Autodesk Inventor part; units mm, degrees
ref_plane "YZ Plane" through (0, 0, 0) normal (1, 0, 0) x (0, 1, 0)
ref_plane "XZ Plane" through (0, 0, 0) normal (0, 1, 0) x (-1, 0, 0)
ref_plane "XY Plane" through (0, 0, 0) normal (0, 0, 1) x (1, 0, 0)
sketch "Sketch1" plane through (0, 0, 0) normal (0, 1, 0) x (-1, 0, 0)
  line L0 (0, 0) -> (254, 0)
  line L1 (254, 0) -> (254, -119.38)
  line L2 (254, -119.38) -> (0, -119.38)
  line L3 (0, -119.38) -> (0, 0)
  line L4 (186.69, 67.31) -> (67.31, 67.31)
  line L5 (67.31, 67.31) -> (67.31, -186.69)
  line L6 (67.31, -186.69) -> (186.69, -186.69)
  line L7 (186.69, -186.69) -> (186.69, 67.31)
  line L8 (186.69, 67.31) -> (254, 0)
  line L9 (67.31, 67.31) -> (0, 0)
  line L10 (186.69, -186.69) -> (254, -119.38)
  line L11 (0, -119.38) -> (67.31, -186.69)
  line L12 (62.2907, -7.1202) -> (161.0967, -7.1202)
  line L13 (164.2717, -10.2952) -> (164.2717, -109.1012)
  line L14 (161.0967, -112.2762) -> (62.2907, -112.2762)
  line L15 (59.1157, -109.1012) -> (59.1157, -10.2952)
  arc A0 (62.2907, -7.1202) -> (59.1157, -10.2952) centre (62.2907, -10.2952) ccw
  arc A1 (164.2717, -10.2952) -> (161.0967, -7.1202) centre (161.0967, -10.2952) ccw
  arc A2 (161.0967, -112.2762) -> (164.2717, -109.1012) centre (161.0967, -109.1012) ccw
  arc A3 (59.1157, -109.1012) -> (62.2907, -112.2762) centre (62.2907, -109.1012) ccw
  line L16 (254, -119.38) -> (127, -119.38)
  line L17 (126.9917, -59.69) -> (127, -119.38)
  point P0 (164.2717, -112.2762)
  point P1 (164.2717, -7.1202)
  point P2 (59.1157, -112.2762)
  point P3 (127, -59.69)
  point P4 (127, -59.69)
  dimension "d0" = 254
  dimension "d1" = 119.38
  dimension "d2" = 119.38
  dimension "d3" = 254
  dimension "d8" = 95.1907
  dimension "d14" = 105.156
  dimension "d15" = 105.156
  dimension "d22" = 3.175
  dimension "d50" = 127
  dimension "d51" = 59.69
extrude "Extrusion1" add sketch "Sketch1" along normal blind 25.4
sketch "Sketch3" plane through (0, 0, 0) normal (0, -1, 0) x (1, 0, 0)
  line L0 (-80.7772, -112.268) -> (-173.2332, -112.268)
  line L1 (-179.5832, -105.918) -> (-179.5832, -13.462)
  line L2 (-173.2332, -7.112) -> (-80.7772, -7.112)
  line L3 (-74.4272, -13.462) -> (-74.4272, -105.918)
  arc A0 (-80.7772, -112.268) -> (-74.4272, -105.918) centre (-80.7772, -105.918) ccw
  arc A1 (-179.5832, -105.918) -> (-173.2332, -112.268) centre (-173.2332, -105.918) ccw
  arc A2 (-173.2332, -7.112) -> (-179.5832, -13.462) centre (-173.2332, -13.462) ccw
  arc A3 (-74.4272, -13.462) -> (-80.7772, -7.112) centre (-80.7772, -13.462) ccw
  line L4 (-124.213, 67.31) -> (-124.213, -7.112)
  line L5 (-254.0007, -58.0211) -> (-179.5787, -58.0211)
  line L6 (-186.69, 67.31) -> (-67.31, 67.31)
  point P0 (0, 0)
  point P1 (-179.5832, -7.112)
  point P2 (-179.5832, -112.268)
  point P3 (-74.4272, -7.112)
  point P4 (-179.5832, -58.0211)
  dimension "d23" = 105.156
  dimension "d24" = 105.156
  dimension "d42" = 6.35
  dimension "d45" = 74.422
  dimension "d46" = 74.422
extrude "Extrusion2" cut sketch "Sketch3" against normal blind 25.4
equation "\"d0\" = rectangle_L"
equation "\"d1\" = rectangle_01_w"
equation "\"d2\" = rectangle_01_w"
equation "\"d3\" = rectangle_L"
equation "\"d8\" = d9"
equation "\"rectangle_L\" = 254"
equation "\"rectangle_01_w\" = 119.38"
equation "\"d9\" = 95.19071"
equation "\"window_L\" = 105.156"
equation "\"test\" = 74.422"
equation "\"d47\" = 74.422"
equation "\"d48\" = 254"
equation "\"d49\" = 105.156"
equation "\"dot_pos\" = 127"
equation "\"dot_pos_2\" = 59.69"
properties part number "chamber_top"
Read the model definition and answer for the solid it produces. Units are mm, in the model's axes. A direction names the side the tool comes from. Round coordinates to 2 decimals unless told otherwise and drop trailing zeros. Write each loop counter-clockwise with the first axis right and the second up, starting at its lowest first coordinate (ties: lowest second). Pieces come first, ordered by that corner, then holes. Notation, with made-up numbers: (-40, -4) - (-2, -4) arc R18 ccw to (-2, 11) - close; hole circle Ø10 at (81.5, 35). An arc over 180 degrees is marked (long way). One line per question, with ' | ' between items. Start each with the question number.
1. Section C-C (y = 4.75) is taken. Determine the outline of the cut face in (x, z).
2. For a pull along X with two mould halves and no side action, classify faces 1 (the face through (-34, 13, 34)), 2 (the face through (-179.583, 13, -60)), 3 (the face through (-254, 13, -59)) as +X half, -X half, draft (parallel to the pull), parting line (faces both ways), or undercut.
3. Find the intervals of material crossed by probe 1 along Z at (x, y) = (-147, 6.5); probe 2 along X at (y, z) = (6.5, -88.5); probe 3 along Z at (x, y) = (-194, 4), in increasing order. Write a range as [from, to].
4. Section B-B (x = -166) is taken. Determine the outline of the cut face in (y, z), and give its area (3 significant figures).
5. Section D-D (z = -135.5) is taken. Determine the outline of the cut face in (x, y).
6. For faces 4 (the face through (-177.67, 12.52, -8.92)), 5 (the face through (-220, 13, 34)), determine the directions among +Z, -Z, +X, -X, +Y, -Y from which every point of the face is accessible in a straight line to the end or side of a thin tool.
7. Section A-A (z = -52.5) is taken. Determine the outline of the cut face in (x, y), and give its area (3 significant figures).
8. Each of these flat-tipped pins is pushed along its axis until it touches: pin 1 (12 mm diameter, centred on x = -204.5, y = 8.5, fed in from -Z); pin 2 (10 mm diameter, centred on x = -53.5, y = 17.5, fed in from -Z); pin 3 (3 mm diameter, centred on y = 13.5, z = 40.5, fed in from -X). Where does it stop, or does it pass through?
Filled in:
1) outline: (-254, -119.38) - (-186.69, -186.69) - (-67.31, -186.69) - (0, -119.38) - (0, 0) - (-67.31, 67.31) - (-186.69, 67.31) - (-254, 0) - close; hole (-179.58, -105.92) arc R6.35 ccw to (-173.23, -112.27) - (-80.78, -112.27) arc R6.35 ccw to (-74.43, -105.92) - (-74.43, -13.46) arc R6.35 ccw to (-80.78, -7.11) - (-173.23, -7.11) arc R6.35 ccw to (-179.58, -13.46) - close
2) face 1: +X half | face 2: undercut | face 3: -X half
3) probe 1: [-186.69, -112.27], [-7.11, 67.31] | probe 2: [-254, -179.58], [-74.43, 0] | probe 3: [-179.38, 60]
4) outline: (0, -186.69) - (25.4, -186.69) - (25.4, -112.27) - (0, -112.27) - close; (0, -7.11) - (25.4, -7.11) - (25.4, 67.31) - (0, 67.31) - close | area: 3,780 mm²
5) outline: (-237.88, 0) - (-16.12, 0) - (-16.12, 25.4) - (-237.88, 25.4) - close
6) face 4: +Y, -Y | face 5: +Z, -X, +Y, -Y
7) outline: (-254, 0) - (-179.58, 0) - (-179.58, 25.4) - (-254, 25.4) - close; (-74.43, 0) - (0, 0) - (0, 25.4) - (-74.43, 25.4) - close | area: 3,780 mm²
8) pin 1: z = -174.88 | pin 2: z = -177.88 | pin 3: x = -215
